Geometry check sheet. Reference: the model listing, model coordinates, mm. Face numbers are marked on the shaded views. A direction names the side the tool comes from. Round coordinates to 2 decimals unless told otherwise and drop trailing zeros. Order: outer loops, then holes, each group sorted by start corner. A loop starts at its lowest first (then second) coordinate and runs counter-clockwise, first axis right, second up.
(1) Material ranges on line 1 along Z through (x, y) = (132.75, 9); line 2 along Y through (x, z) = (103.5, 15); line 3 along X through (y, z) = (22.5, -20), recorded low to high.
(2) Sectioned sample at D-D (z = -34). Record the boundary of the cut face in (x, y), plus the area to 3 significant figures.
(3) Set-up check for the marked faces 1 and 2: record each of +Z, -Z, +X, -X, +Y, -Y from which the full face is reachable in a straight line by a thin tool's end or side.
(4) Sectioned sample at A-A (y = 16). Record the boundary of the cut face in (x, z).
(5) Sectioned sample at B-B (z = 14). Record the boundary of the cut face in (x, y).
(6) Go/stop test with flat-tipped pins: pin 1 (3 mm diameter, centred on x = 97, z = 12.5, fed in from +Y); pin 2 (1 mm diameter, centred on y = 12, z = 1.5, fed in from -X); pin 3 (6 mm diameter, centred on y = 8.5, z = -22.5, fed in from -X). Record where each tip stops, or that it passes through.
(7) Release check for a two-part mould opening along Z. For the marked faces 3, 4 and 5 record: +Z half, -Z half, draft (parallel to the pull), parting line (faces both ways), or undercut.
(8) Sectioned sample at C-C (x = -144). Record the boundary of the cut face in (y, z), plus the area to 3 significant figures.
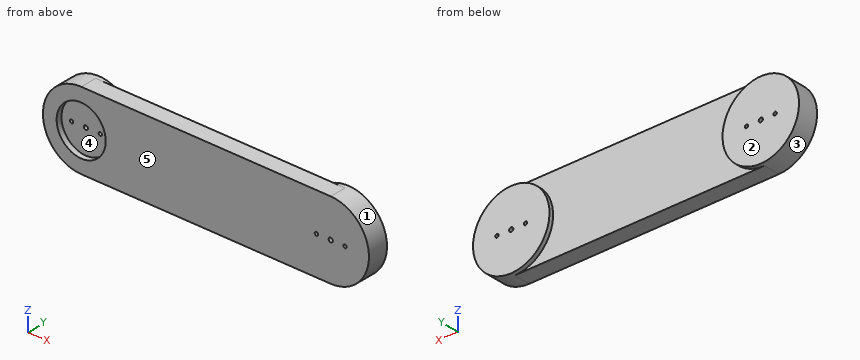
from build123d import *

# Parameters (mm, degrees)
SKETCH_1_W          = 300
SKETCH_1_H          = 92
EXTRUDE_1_DEPTH     = 20
SKETCH_2_R          = 46
EXTRUDE_2_DEPTH     = 25
SKETCH_3_R          = 2.5
SKETCH_3_R_2        = 2
CUT_EXTRUDE_1_DEPTH = 203.871880752
SKETCH_4_R          = 2.5
SKETCH_4_R_2        = 2
CUT_EXTRUDE_2_DEPTH = 203.871880752
SKETCH_5_R          = 29.5
CUT_EXTRUDE_3_DEPTH = 6.6


with BuildPart() as part:
    # 草图1 → 凸台-拉伸1 (new body)
    with BuildSketch(Plane(origin=(0, 0, 0), x_dir=(1, 0, 0), z_dir=(0, 1, 0))):
        Rectangle(SKETCH_1_W, SKETCH_1_H)
    extrude(amount=EXTRUDE_1_DEPTH)

    # 草图2 → 凸台-拉伸2 (add)
    with BuildSketch(Plane.XZ):
        with Locations(Location((-150, 0, 0), (0, 0, 270))):
            Circle(SKETCH_2_R)
        with Locations(Location((150, 0, 0), (0, 0, 270))):
            Circle(SKETCH_2_R)
    extrude(amount=-EXTRUDE_2_DEPTH)

    # 草图3 → 切除-拉伸1 (cut, through all)
    with BuildSketch(Plane(origin=(0, 25, 0), x_dir=(1, 0, 0), z_dir=(0, 1, 0))):
        with Locations(Location((150, 0, 0), (0, 0, 270))):
            Circle(SKETCH_3_R)
        with Locations(Location((167.25, 0, 0), (0, 0, 270))):
            Circle(SKETCH_3_R_2)
        with Locations(Location((132.75, 0, 0), (0, 0, 270))):
            Circle(SKETCH_3_R_2)
    extrude(amount=-CUT_EXTRUDE_1_DEPTH, mode=Mode.SUBTRACT)

    # 草图4 → 切除-拉伸2 (cut, through all)
    with BuildSketch(Plane(origin=(0, 25, 0), x_dir=(1, 0, 0), z_dir=(0, 1, 0))):
        with Locations(Location((-150, 0, 0), (0, 0, 270))):
            Circle(SKETCH_4_R)
        with Locations(Location((-132.75, 0, 0), (0, 0, 270))):
            Circle(SKETCH_4_R_2)
        with Locations(Location((-167.25, 0, 0), (0, 0, 270))):
            Circle(SKETCH_4_R_2)
    extrude(amount=-CUT_EXTRUDE_2_DEPTH, mode=Mode.SUBTRACT)

    # 草图5 → 切除-拉伸3 (cut)
    with BuildSketch(Plane.XZ):
        with Locations(Location((-150, 0, 0), (0, 0, 270))):
            Circle(SKETCH_5_R)
    extrude(amount=-CUT_EXTRUDE_3_DEPTH, mode=Mode.SUBTRACT)


solid = part.part
Answer below:
1. line 1: z = -46 to -2, 2 to 46
1. line 2: y = 0 to 20
1. line 3: x = -191.42 to -108.58, 108.58 to 191.42
2. outline: (-180.98, 0) - (180.98, 0) - (180.98, 25) - (119.02, 25) - (119.02, 20) - (-119.02, 20) - (-119.02, 25) - (-180.98, 25) - close
2. area: 7,860 mm2
3. face 1: +Y
3. face 2: +Z, -Z, +X, -X, +Y
4. outline: (-150, -46) - (150, -46) arc R46 ccw to (150, 46) - (-150, 46) arc R46 ccw to start; hole circle Ø4 at (-167.25, 0); hole circle Ø5 at (-150, 0); hole circle Ø4 at (-132.75, 0); hole circle Ø4 at (132.75, 0); hole circle Ø5 at (150, 0); hole circle Ø4 at (167.25, 0)
5. outline: (-193.82, 0) - (-175.97, 0) - (-175.97, 6.6) - (-124.03, 6.6) - (-124.03, 0) - (193.82, 0) - (193.82, 25) - (106.18, 25) - (106.18, 20) - (-106.18, 20) - (-106.18, 25) - (-193.82, 25) - close
6. pin 1: stops at y = 20
6. pin 2: stops at x = -195.99
6. pin 3: stops at x = -191.66
7. face 3: parting line
7. face 4: undercut
7. face 5: draft
8. outline: (0, -46) - (20, -46) - (20, -45.61) - (25, -45.61) - (25, 45.61) - (20, 45.61) - (20, 46) - (0, 46) - (0, 28.88) - (6.6, 28.88) - (6.6, -28.88) - (0, -28.88) - close
8. area: 1,910 mm2
